The model under review builds one solid part; all positions refer to its coordinate system, in mm. Face numbers are marked on the shaded views. A direction names the side the tool comes from. Coordinates: 2 decimals unless noted, no trailing zeros. Order: outer loops, then holes, each group sorted by start corner. A loop starts at its lowest first (then second) coordinate and runs counter-clockwise, first axis right, second up. Notation, with made-up numbers: (46, 66) - (72, 66) arc R18 cw to (72, 80) - close; hole circle Ø8 at (83, 46.5). An arc over 180 degrees is marked (long way). Answer in a Markdown table with one row per item.
```python
from build123d import *

# Parameters (mm, degrees)
SKETCH1_W           = 74.22368895
SKETCH1_H           = 68
SKETCH1_W_2         = 37.111844475
SKETCH1_H_2         = 52
SKETCH1_H_3         = 58
BOSS_EXTRUDE1_DEPTH = 70
SKETCH2_R           = 27.5
CUT_EXTRUDE1_DEPTH  = 70
FILLET1_R           = 19
SKETCH3_W           = 33.111844475
SKETCH3_H           = 64.288874977
CUT_EXTRUDE2_DEPTH  = 58
SKETCH5_W           = 50
SKETCH5_H           = 40
CUT_EXTRUDE3_DEPTH  = 58
SKETCH7_W           = 29.516350972
SKETCH7_H           = 18.630296647
CUT_EXTRUDE5_DEPTH  = 58
SKETCH8_W           = 33.111844475
SKETCH8_H           = 2
CUT_EXTRUDE6_DEPTH  = 58
SKETCH9_W           = 1.55
SKETCH9_H           = 66.288874977
BOSS_EXTRUDE2_DEPTH = 58
SKETCH10_W          = 30.011844475
SKETCH10_H          = 0.145
BOSS_EXTRUDE3_DEPTH = 58


with BuildPart() as part:
    # Sketch1 → Boss-Extrude1 (new body)
    with BuildSketch(Plane(origin=(0, 0, 0), x_dir=(1, 0, 0), z_dir=(0, 1, 0))):
        with Locations((-37.111844475, -34)):
            Rectangle(SKETCH1_W, SKETCH1_H)
        with Locations((-37.111844475, -94)):
            Rectangle(SKETCH1_W_2, SKETCH1_H_2)
        with Locations((-37.111844475, -149)):
            Rectangle(SKETCH1_W_2, SKETCH1_H_3)
    extrude(amount=-BOSS_EXTRUDE1_DEPTH)

    # Sketch2 → Cut-Extrude1 (cut)
    with BuildSketch(Plane(origin=(0, 0, 0), x_dir=(1, 0, 0), z_dir=(0, 1, 0))):
        with Locations(Location((-37.111844475, -34, 0), (0, 0, 270))):
            Circle(SKETCH2_R)
    extrude(amount=-CUT_EXTRUDE1_DEPTH, mode=Mode.SUBTRACT)

    # Fillet1
    # the kernel refuses this fillet: 19 mm, written as the material it takes off along each edge
    with BuildSketch(Plane(origin=(0, 47.487024211, 68), x_dir=(0, 0, -1), z_dir=(0, -1, 0))) as fillet1_piece_1:
        with BuildLine():
            CenterArc((18.994809684, -19), FILLET1_R, 90, 88.660731648)
            Line((0, -18.555922237), (-0.379896194, -18.547040682))
            ThreePointArc((-0.379896194, -18.547040682), (-0.38, -9.277961119), (-0.38, 0))
            Line((-0.38, 0), (0, 0.38))
            Line((0, 0.38), (18.994809684, 0.38))
            Line((18.994809684, 0.38), (18.994809684, 0))
        make_face()
    extrude(amount=164.974048421, mode=Mode.SUBTRACT)
    with BuildSketch(Plane(origin=(0, 47.5, 0), x_dir=(-1, 0, 0), z_dir=(0, -1, 0))) as fillet1_piece_2:
        with BuildLine():
            CenterArc((FILLET1_R, -FILLET1_R), FILLET1_R, 90, 90)
            Line((0, -FILLET1_R), (-FILLET1_R * 0.02, -FILLET1_R))
            Line((-FILLET1_R * 0.02, -FILLET1_R), (-FILLET1_R * 0.02, FILLET1_R * 0.02))
            Line((-FILLET1_R * 0.02, FILLET1_R * 0.02), (FILLET1_R, FILLET1_R * 0.02))
            Line((FILLET1_R, FILLET1_R * 0.02), (FILLET1_R, 0))
        make_face()
    extrude(amount=165, mode=Mode.SUBTRACT)
    with BuildSketch(Plane(origin=(-74.22368895, 47.487024211, 68), x_dir=(0, 0, -1), z_dir=(0, -1, 0))) as fillet1_piece_3:
        with BuildLine():
            CenterArc((18.994809684, 19), FILLET1_R, 181.339268352, 88.660731648)
            Line((0, 18.555922237), (-0.379896194, 18.547040682))
            ThreePointArc((-0.379896194, 18.547040682), (-0.38, 9.277961119), (-0.38, 0))
            Line((-0.38, 0), (0, -0.38))
            Line((0, -0.38), (18.994809684, -0.38))
            Line((18.994809684, -0.38), (18.994809684, 0))
        make_face()
    extrude(amount=164.974048421, mode=Mode.SUBTRACT)
    with BuildSketch(Plane(origin=(-74.22368895, 47.5, 0), x_dir=(1, 0, 0), z_dir=(0, -1, 0))) as fillet1_piece_4:
        with BuildLine():
            CenterArc((FILLET1_R, FILLET1_R), FILLET1_R, 180, 90)
            Line((0, FILLET1_R), (-FILLET1_R * 0.02, FILLET1_R))
            Line((-FILLET1_R * 0.02, FILLET1_R), (-FILLET1_R * 0.02, -FILLET1_R * 0.02))
            Line((-FILLET1_R * 0.02, -FILLET1_R * 0.02), (FILLET1_R, -FILLET1_R * 0.02))
            Line((FILLET1_R, -FILLET1_R * 0.02), (FILLET1_R, 0))
        make_face()
    extrude(amount=165, mode=Mode.SUBTRACT)

    # Sketch3 → Cut-Extrude2 (cut)
    with BuildSketch(Plane.XY.offset(178)):
        with Locations((-37.111844475, -35.855562511)):
            Rectangle(SKETCH3_W, SKETCH3_H)
    extrude(amount=-CUT_EXTRUDE2_DEPTH, mode=Mode.SUBTRACT)

    # Sketch5 → Cut-Extrude3 (cut)
    with BuildSketch(Plane.ZY.offset(55.667766712)):
        with Locations((93, -50)):
            Rectangle(SKETCH5_W, SKETCH5_H)
    extrude(amount=-CUT_EXTRUDE3_DEPTH, mode=Mode.SUBTRACT)

    # Sketch7 → Cut-Extrude5 (cut)
    with BuildSketch(Plane(origin=(0, 0, 118), x_dir=(-1, 0, 0), z_dir=(0, 0, -1))):
        with Locations((37.314097723, -50.684851677)):
            Rectangle(SKETCH7_W, SKETCH7_H)
    extrude(amount=-CUT_EXTRUDE5_DEPTH, mode=Mode.SUBTRACT)

    # Sketch8 → Cut-Extrude6 (cut)
    with BuildSketch(Plane.XY.offset(178)):
        with Locations((-37.111844475, -2.711125023)):
            Rectangle(SKETCH8_W, SKETCH8_H)
    extrude(amount=-CUT_EXTRUDE6_DEPTH, mode=Mode.SUBTRACT)

    # Sketch9 → Boss-Extrude2 (add)
    with BuildSketch(Plane.XY.offset(178)):
        with Locations((-52.892766712, -34.855562511)):
            Rectangle(SKETCH9_W, SKETCH9_H)
        with Locations((-21.330922237, -34.855562511)):
            Rectangle(SKETCH9_W, SKETCH9_H)
    extrude(amount=-BOSS_EXTRUDE2_DEPTH)

    # Sketch10 → Boss-Extrude3 (add)
    with BuildSketch(Plane.XY.offset(178)):
        with Locations((-37.111844475, -67.9275)):
            Rectangle(SKETCH10_W, SKETCH10_H)
        with Locations((-37.111844475, -1.783625023)):
            Rectangle(SKETCH10_W, SKETCH10_H)
    extrude(amount=-BOSS_EXTRUDE3_DEPTH)


solid = part.part
```
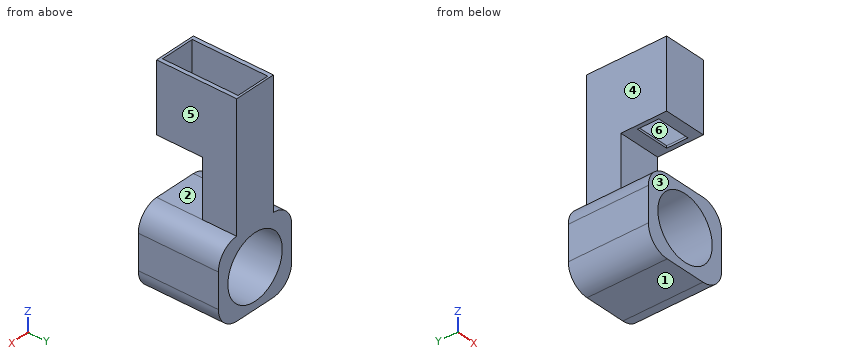
Item 1: We need section D-D, the plane x = -40.5. Write out the cut boundary in (y, z) (3 decimals), then the cut area to 3 significant figures.
Check values:
| item | result |
|---|---|
| outline | (-70, 0) - (0, 0) - (0, 6.71) - (-70, 6.71) - close; (-70, 61.29) - (0, 61.29) - (0, 178) - (-1.856, 178) - (-1.856, 120) - (-41.37, 120) - (-41.37, 118) - (-30, 118) - (-30, 68) - (-70, 68) - close; (-70, 118) - (-60, 118) - (-60, 120) - (-67.855, 120) - (-67.855, 178) - (-70, 178) - close |
| area | 2,770 mm^2 |
Item 2: We need section C-C, the plane z = 144.5. Write out the cut boundary in (x, y) (3 decimals).
Check values:
| item | result |
|---|---|
| outline | (-55.668, -70) - (-18.556, -70) - (-18.556, 0) - (-55.668, 0) - close; hole (-52.118, -67.855) - (-22.106, -67.855) - (-22.106, -1.856) - (-52.118, -1.856) - close |
Item 3: Mouldability with a two-part tool opening along Z and no side actions: class the marked faces 1, 2 and 3 as +Z half, -Z half, draft (parallel to the pull), parting line (faces both ways), or undercut.
Check values:
| item | result |
|---|---|
| face 1 | -Z half |
| face 2 | undercut |
| face 3 | draft |
Item 4: We need section B-B, the plane y = -58. Write out the cut boundary in (x, z), then the cut area to 3 significant figures.
Check values:
| item | result |
|---|---|
| outline | (-74.22, 19) arc R19 ccw to (-55.22, 0) - (-19, 0) arc R19 ccw to (0, 19) - (0, 49.01) arc R19 ccw to (-18.56, 68) - (-55.67, 68) arc R19 ccw to (-74.22, 49.01) - close; (-55.67, 118) - (-52.07, 118) - (-52.07, 120) - (-52.12, 120) - (-52.12, 178) - (-55.67, 178) - close; (-22.56, 118) - (-18.56, 118) - (-18.56, 178) - (-22.11, 178) - (-22.11, 120) - (-22.56, 120) - close; hole circle Ø55 at (-37.11, 34) |
| area | 2,790 mm^2 |
Item 5: Clearance check with flat-ended pins moving along their axes: pin 1 Ø8 at (x, y) = (-11.5, -21) entering from +Z; pin 2 Ø10 at (y, z) = (-19, 113.5) entering from -X; pin 3 Ø1 at (y, z) = (-55, 119) entering from +X. State where each tip first meets the part, or that it passes through.
Check values:
| item | result |
|---|---|
| pin 1 | z = 67.68 |
| pin 2 | x = -55.67 |
| pin 3 | x = -18.56 |
Item 6: We need section A-A, the plane z = 34. Write out the cut boundary in (x, y), then the cut area to 3 significant figures.
Check values:
| item | result |
|---|---|
| outline | (-74.22, -70) - (-64.61, -70) - (-64.61, 0) - (-74.22, 0) - close; (-9.61, -70) - (0, -70) - (0, 0) - (-9.61, 0) - close |
| area | 1,350 mm^2 |
Item 7: Tool access review of the marked faces 4, 5 and 6: name each direction out of +Z, -Z, +X, -X, +Y, -Y from which nothing blocks a thin tool from reaching the whole face with its end or side.
Check values:
| item | result |
|---|---|
| face 4 | +Z, -X, +Y, -Y |
| face 5 | +Z, +X, +Y, -Y |
| face 6 | +Z |
Item 8: To check wall thickness, follow line 1 (X direction, y = -7, z = 145.5); line 2 (X direction, y = -27, z = 34); line 3 (Z direction, x = -25.5, y = -65.5). State the ranges of each line that lie inside material, in increasing order. Write a range as from..to.
Check values:
| item | result |
|---|---|
| line 1 | -55.67..-52.12, -22.11..-18.56 |
| line 2 | -74.22..-64.61, -9.61..0 |
| line 3 | 0..9.07, 58.93..68, 118..120 |
